from build123d import *

# Parameters (mm, degrees)
F1_DEPTH = 12.7
F2_R     = 5.08
F3_R     = 5.08


with BuildPart() as f1:
    # F0 (on Front) → F1 (new body, symmetric)
    with BuildSketch(Plane.XZ):
        with BuildLine():
            Line((-24.244117, 34.463618), (-58.59901, 34.463618))
            Line((-58.59901, 34.463618), (-58.59901, -42.943612))
            Line((-58.59901, -42.943612), (60.990814, -42.943612))
            Line((60.990814, -42.943612), (60.990814, 10.545651))
            Line((60.990814, 10.545651), (0, 10.545651))
            ThreePointArc((0, 10.545651), (-17.028258, 17.531533), (-24.244117, 34.463618))
        make_face()
    extrude(amount=F1_DEPTH, both=True)

    # F2
    f2_edges = [f1.edges().sort_by_distance(p)[0] for p in [
        (-58.59901, 0, 34.463618),
        (60.990814, 0, 10.545651),
        (60.990814, 0, -42.943612),
    ]]
    fillet(f2_edges, radius=F2_R)

    # F3
    f3_edges = [f1.edges().sort_by_distance(p)[0] for p in [
        (-58.59901, 0, -42.943612),
        (-24.244117, 0, 34.463618),
    ]]
    fillet(f3_edges, radius=F3_R)


solid = f1.part
Build history of the part. All positions in model axes, mm. A direction names the side the tool comes from. Round coordinates to 2 decimals unless told otherwise and drop trailing zeros. Write each loop counter-clockwise with the first axis right and the second up, starting at its lowest first coordinate (ties: lowest second). Pieces come first, ordered by that corner, then holes. Notation, with made-up numbers: (-18.75, 48.5) -> (39.25, 48.5) arc R30 ccw to (39.25, 77.5) -> close; hole circle Ø6 at (49.5, 72.5). An arc over 180 degrees is marked (long way). Use one line per item in the form item = value.
Q1. Tool access for faces 1 (the flat face through (-41, 0, 34.464)), 2 (the flat face through (28, 0, 10.546)): list every direction of +Z, -Z, +X, -X, +Y, -Y with a clear straight run to the whole face (end or side of a thin tool).
Conclusion:
face_1 = +Z, +X, -X, +Y, -Y
face_2 = +Z, +X, +Y, -Y
Q2. Drill centre lines: L1, parallel to Z at x = 10, y = 6.75; L2, parallel to X at y = -7.5, z = 25.5; L3, parallel to Z at x = -3.5, y = -0.75. Where is each one in solid material? Low to high.
Conclusion:
L1 = -42.94 to 10.55
L2 = -58.6 to -22.4
L3 = -42.94 to 10.8
Q3. Band-saw the part on C-C, the plane z = 12. Write the cut outline in (x, y).
Conclusion:
outline = (-58.6, -12.7) -> (-8.27, -12.7) -> (-8.27, 12.7) -> (-58.6, 12.7) -> close
Q4. Band-saw the part on B-B, the plane x = 15.5. Write the cut outline in (y, z), then the cut area to 3 significant figures.
Conclusion:
outline = (-12.7, -42.94) -> (12.7, -42.94) -> (12.7, 10.55) -> (-12.7, 10.55) -> close
area = 1,360 mm²
Q5. Drop flat-ended pins along their axis: P1, Ø2, axis at x = 7, y = 2.5, coming from the +Z side; P2, Ø4, axis at y = -1, z = 23, coming from the +X side. Give the stop position or say it passes through.
Conclusion:
P1 = 10.55
P2 = -19.94
Q6. Band-saw the part on A-A, the plane y = 0. Write the cut outline in (x, z), then the cut area to 3 significant figures.
Conclusion:
outline = (-58.6, -37.86) arc R5.08 ccw to (-53.52, -42.94) -> (55.91, -42.94) arc R5.08 ccw to (60.99, -37.86) -> (60.99, 5.47) arc R5.08 ccw to (55.91, 10.55) -> (0, 10.55) arc R24.25 cw to (-23.83, 30.32) arc R5.08 ccw to (-28.82, 34.46) -> (-53.52, 34.46) arc R5.08 ccw to (-58.6, 29.38) -> close
area = 7,320 mm²
